Read the model definition and answer for the solid it produces. Units are mm, in the model's axes. A direction names the side the tool comes from. Coordinates: 2 decimals unless noted, no trailing zeros. Write each loop counter-clockwise with the first axis right and the second up, starting at its lowest first coordinate (ties: lowest second). Pieces come first, ordered by that corner, then holes. Notation, with made-up numbers: (-4.5, -2) -> (52.5, -2) arc R4 ccw to (52.5, 4) -> close; hole circle Ø3 at (1, 85). An arc over 180 degrees is marked (long way). One line per item, written item: value. Start each with the question number.
from build123d import *

# Parameters (mm, degrees)
BASE_FLANGE1_DEPTH = 500
SKETCH4_R          = 2.55
CUT_EXTRUDE1_DEPTH = 501.278732308


# Sheet-metal steps are written as plain solids
with BuildPart() as part:
    # Sketch1 → Base-Flange1 (new body)
    with BuildSketch(Plane(origin=(0, 0, 0), x_dir=(0, 0, -1), z_dir=(1, 0, 0))):
        with BuildLine():
            Line((4.05, -6), (4.05, 4.2634))
            ThreePointArc((4.05, 4.2634), (3.541361636, 5.491361636), (2.3134, 6))
            Line((2.3134, 6), (-3.3134, 6))
            ThreePointArc((-3.3134, 6), (-3.834254855, 6.215745145), (-4.05, 6.7366))
            Line((-4.05, 6.7366), (-4.05, 14))
            Line((-4.05, 14), (-5.05, 14))
            Line((-5.05, 14), (-5.05, 6.7366))
            ThreePointArc((-5.05, 6.7366), (-4.541361636, 5.508638364), (-3.3134, 5))
            Line((-3.3134, 5), (2.3134, 5))
            ThreePointArc((2.3134, 5), (2.834254855, 4.784254855), (3.05, 4.2634))
            Line((3.05, 4.2634), (3.05, -6))
            Line((3.05, -6), (4.05, -6))
        make_face()
    extrude(amount=BASE_FLANGE1_DEPTH)

    # Sketch4 → Cut-Extrude1 (cut, through all)
    with BuildSketch(Plane(origin=(0, 0, -4.05), x_dir=(-1, 0, 0), z_dir=(0, 0, -1))):
        with Locations((-420, -0.729372)):
            Circle(SKETCH4_R)
        with Locations((-80, -0.138928)):
            Circle(SKETCH4_R)
    extrude(amount=-CUT_EXTRUDE1_DEPTH, mode=Mode.SUBTRACT)


solid = part.part
1. A cutting plane is placed at A-A on x = 245.5. Give the vertices of the cut face in (y, z).
2. Given pin 1 (1.5 mm diameter, centred on x = 266.5, y = 1.5, fed in from +Z); pin 2 (1 mm diameter, centred on x = 422.5, z = -1.5, fed in from +Y); pin 3 (3 mm diameter, centred on x = 153.5, z = 0.5, fed in from -Y), each flat-ended and moving along its own axis, determine where each tip first touches the part or whether it passes through.
3. A tool of negligible diameter and unlimited length cuts with its end or side. For faces 1 (the face through (246, -1, -3.05)), 2 (the face through (0, 5.5, 0.2)), from which of +Z, -Z, +X, -X, +Y, -Y can it reach the whole face along a straight path? Write none if from no direction.
4. A cutting plane is placed at B-B on z = 0. Give the vertices of the cut face in (x, y).
5. Find the intervals of material crossed by probe 1 along Z at (x, y) = (251.5, 3.5); probe 2 along Y at (x, z) = (345.5, 2.75); probe 3 along Z at (x, y) = (339, 7.5), in increasing order. Write a range as from..to.
Derived:
1. outline: (-6, -4.05) -> (4.26, -4.05) arc R1.74 ccw to (6, -2.31) -> (6, 3.31) arc R0.74 cw to (6.74, 4.05) -> (14, 4.05) -> (14, 5.05) -> (6.74, 5.05) arc R1.74 ccw to (5, 3.31) -> (5, -2.31) arc R0.74 cw to (4.26, -3.05) -> (-6, -3.05) -> close
2. pin 1: stops at z = -3.05
2. pin 2: stops at y = 6
2. pin 3: stops at y = 5
3. face 1: +Z, +X, -X, -Y
3. face 2: +Z, -Z, -X, +Y, -Y
4. outline: (0, 5) -> (500, 5) -> (500, 6) -> (0, 6) -> close
5. probe 1: z = -4.05..-3.05
5. probe 2: y = 5..6
5. probe 3: z = 4.05..5.05
